Job drawing, mm, ordinate dimensions from the low corner. One solid piece. A direction names the side the tool comes from. Coordinates: 2 decimals unless noted, no trailing zeros. Write each loop counter-clockwise with the first axis right and the second up, starting at its lowest first coordinate (ties: lowest second). Pieces come first, ordered by that corner, then holes. Notation, with made-up numbers: (16, -12) - (53, -12) arc R13 ccw to (53, 3) - close; hole circle Ø3 at (-23.75, 57.5). An arc over 180 degrees is marked (long way). Use one line per item in the form item = value. Start each with the question number.
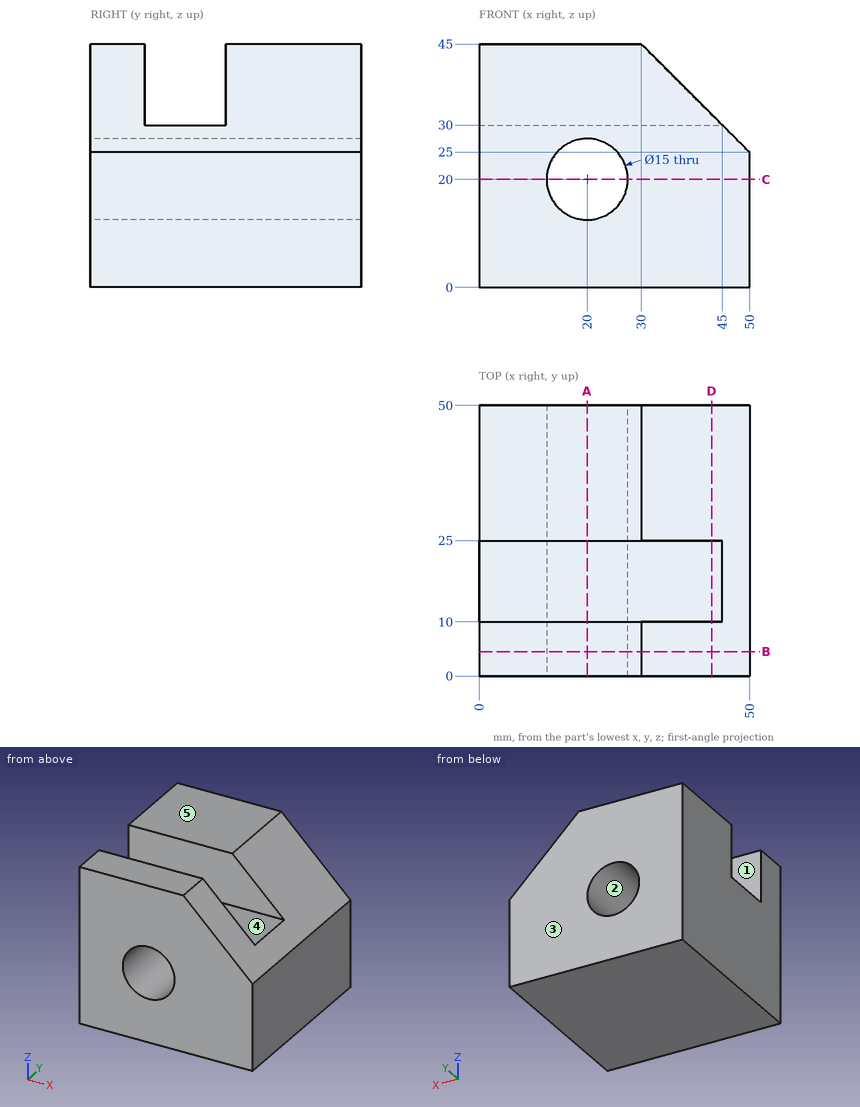
Q1. Slice it at C-C (z = 20). List the corners of the cut face in (x, y).
Q2. Slice it at A-A (x = 20). List the corners of the cut face in (y, z).
Q3. Mould opens along Y. For the marked faces 3, 4 and 5 say: released by +Y, released by -Y, zero draft, split by the parting line, or undercut.
Q4. Pin check, flat tips, straight feed: P1, Ø1.5, axis at y = 32, z = 33.5, coming from the +X side; P2, Ø5, axis at x = 43, y = 31, coming from the +Z side; P3, Ø6, axis at x = 18.5, y = 19.5, coming from the +Z side. Stop position of each tip, or through.
Q5. Slice it at B-B (y = 4.5). List the corners of the cut face in (x, z), plus the area to 3 significant figures.
Q6. Which spindle directions (+Z, -Z, +X, -X, +Y, -Y) get a long thin tool onto all of the face, cutting with end or side? Do the marked faces 1 and 2. Say none if no direction does.
Q7. Slice it at D-D (x = 43). List the corners of the cut face in (y, z), plus the area to 3 significant figures.
Q8. Drill centre lines: probe 1 along Y at (x, z) = (4.5, 31); probe 2 along Z at (x, y) = (20, 21); probe 3 along Z at (x, y) = (20, 35). Where is each one in solid material? Low to high.
Solution:
q1.outline = (0, 0) - (12.5, 0) - (12.5, 50) - (0, 50) - close; (27.5, 0) - (50, 0) - (50, 50) - (27.5, 50) - close
q2.outline = (0, 0) - (50, 0) - (50, 12.5) - (0, 12.5) - close; (0, 27.5) - (50, 27.5) - (50, 45) - (25, 45) - (25, 30) - (10, 30) - (10, 45) - (0, 45) - close
q3.face_3 = released by +Y
q3.face_4 = undercut
q3.face_5 = zero draft
q4.P1 = 42.25
q4.P2 = 34.5
q4.P3 = 30
q5.outline = (0, 0) - (50, 0) - (50, 25) - (30, 45) - (0, 45) - close; hole circle Ø15 at (20, 20)
q5.area = 1,870 mm2
q6.face_1 = +Z, +X, -X
q6.face_2 = +Y, -Y
q7.outline = (0, 0) - (50, 0) - (50, 32) - (25, 32) - (25, 30) - (10, 30) - (10, 32) - (0, 32) - close
q7.area = 1,570 mm2
q8.probe_1 = 0 to 10, 25 to 50
q8.probe_2 = 0 to 12.5, 27.5 to 30
q8.probe_3 = 0 to 12.5, 27.5 to 45
